Can you work these out from the drawing? Everything is in mm from the part's minimum corner. Give positions to 0.01 mm unless a question says otherwise; leave off trailing zeros. Write each loop counter-clockwise with the first axis right and the second up, starting at its lowest first coordinate (ties: lowest second). Pieces come first, ordered by that corner, then holes. Notation, with made-up numbers: (-19.5, 38.5) - (32.5, 38.5) arc R36 ccw to (32.5, 73.5) - close; hole circle Ø7 at (-16.75, -0.5). An arc over 180 degrees is marked (long way). Write each question's results on one line, items separated by ' | '. Start each with the question number.
Item 1: Suppose I cut it at C-C on z = 28. List the corners of the cut face in (x, y) for me.
Item 2: Please list where these lines run through material, in increasing order: line 1 along Y through (x, z) = (19.05, 55.5); line 2 along X through (y, z) = (24, 49.5).
Item 3: Suppose I cut it at B-B on y = 20.5. List the corners of the cut face in (x, z) for me, then the cut area to 3 significant figures.
Item 4: We'd pull the mould along X, two halves only. Please class the marked faces 1, 2, 3 and 4: +X half, -X half, draft (parallel to the pull), parting line (faces both ways), or undercut.
Item 5: Suppose I cut it at A-A on x = 19.05. List the corners of the cut face in (y, z) for me, then the cut area to 3 significant figures.
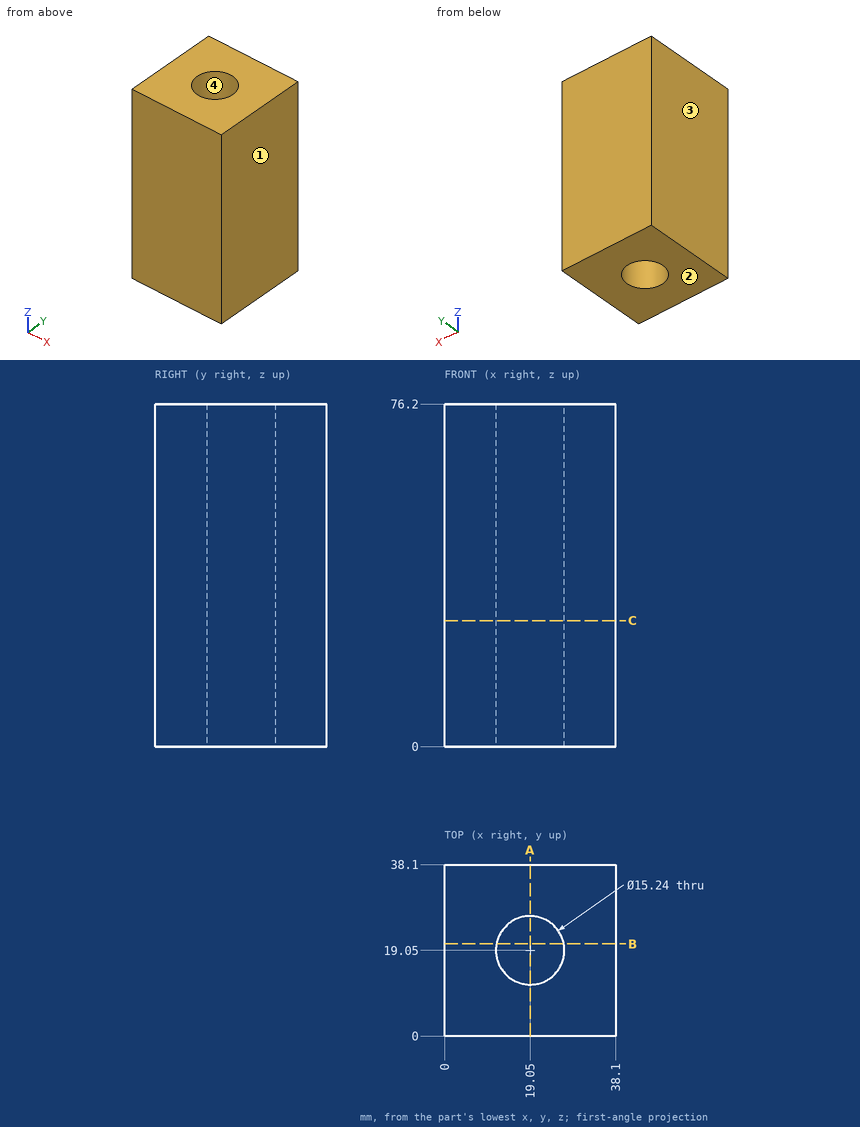
Checked values:
1) outline: (0, 0) - (38.1, 0) - (38.1, 38.1) - (0, 38.1) - close; hole circle Ø15.24 at (19.05, 19.05)
2) line 1: y = 0 to 11.43, 26.67 to 38.1 | line 2: x = 0 to 13.26, 24.84 to 38.1
3) outline: (0, 0) - (11.57, 0) - (11.57, 76.2) - (0, 76.2) - close; (26.53, 0) - (38.1, 0) - (38.1, 76.2) - (26.53, 76.2) - close | area: 1,760 mm^2
4) face 1: +X half | face 2: draft | face 3: -X half | face 4: undercut
5) outline: (0, 0) - (11.43, 0) - (11.43, 76.2) - (0, 76.2) - close; (26.67, 0) - (38.1, 0) - (38.1, 76.2) - (26.67, 76.2) - close | area: 1,740 mm^2
